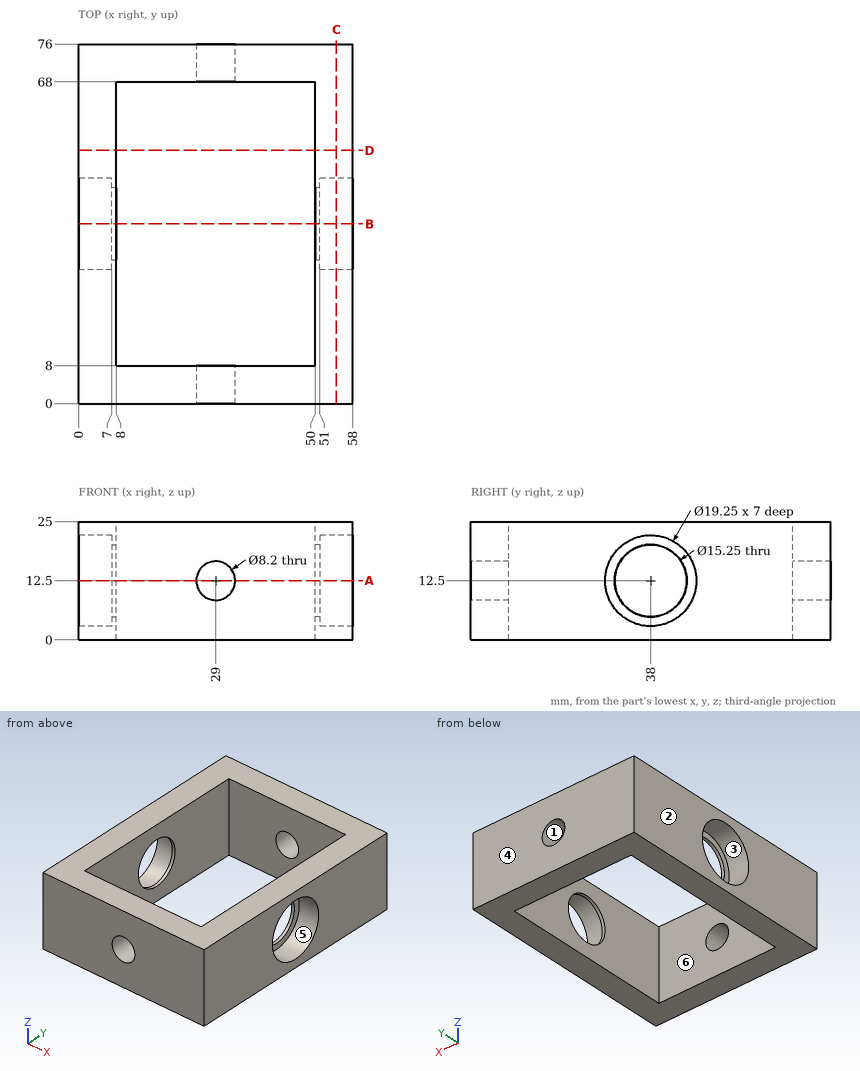
For this review, use the dimensioned drawing (mm, ordinates from the lowest corner) and the shaded views. A direction names the side the tool comes from. Coordinates: 2 decimals unless noted, no trailing zeros. Loops run counter-clockwise (first coordinate to the right, second up) from the corner with the lowest first, then second, coordinate; pieces in that order, holes last. Notation, with made-up numbers: (62, -35) - (66, -35) arc R16 ccw to (66, -4) - close; hole circle Ø5 at (82, -31). An arc over 180 degrees is marked (long way). Use one line per item in the form item = value. Start each with the question number.
1) For pin 1 (6 mm diameter, centred on y = 35, z = 8, fed in from +X); pin 2 (9 mm diameter, centred on y = 38, z = 12.5, fed in from -X), all flat-tipped, find the tip position at first contact; note any pin that passes through.
2) Take a section at A-A (z = 12.5). State how many separate pieces and enclosed holes the cut face has, plus the area to 3 significant figures.
3) To check wall thickness, follow probe 1 along X at (y, z) = (60.5, 3.5); probe 2 along Y at (x, z) = (44, 12.75); probe 3 along Z at (x, y) = (29, 3). State the ranges of each line that lie inside material, in increasing order. Write a range as from..to.
4) Take a section at B-B (y = 38). State the section outline as (x, z) points (3 decimals), plus the area to 3 significant figures.
5) Draft analysis for pull direction X (two halves, no side actions). For the marked faces 1, 2 and 3, state which applies: released by +X, released by -X, zero draft, split by the parting line, or undercut.
6) Take a section at D-D (y = 53.5). State the section outline as (x, z) points, plus the area to 3 significant figures.
7) Take a section at C-C (x = 54.5). State the section outline as (y, z) points (3 decimals).
8) For the marked faces 4, 5 and 6, list the 3-axis set-ups (+Z, -Z, +X, -X, +Y, -Y) from which the entire face can be reached by the end or side of a thin tool; tool diameter is ignored.
From the geometry:
q1.pin_1 = 51
q1.pin_2 = through
q2.separate_pieces = 4
q2.enclosed_holes = 0
q2.area = 1,460 mm2
q3.probe_1 = 0..8, 50..58
q3.probe_2 = 0..8, 68..76
q3.probe_3 = 0..8.4, 16.6..25
q4.outline = (0, 0) - (8, 0) - (8, 4.875) - (7, 4.875) - (7, 2.875) - (0, 2.875) - close; (0, 22.125) - (7, 22.125) - (7, 20.125) - (8, 20.125) - (8, 25) - (0, 25) - close; (50, 0) - (58, 0) - (58, 2.875) - (51, 2.875) - (51, 4.875) - (50, 4.875) - close; (50, 20.125) - (51, 20.125) - (51, 22.125) - (58, 22.125) - (58, 25) - (50, 25) - close
q4.area = 100 mm2
q5.face_1 = undercut
q5.face_2 = released by -X
q5.face_3 = zero draft
q6.outline = (0, 0) - (8, 0) - (8, 25) - (0, 25) - close; (50, 0) - (58, 0) - (58, 25) - (50, 25) - close
q6.area = 400 mm2
q7.outline = (0, 0) - (76, 0) - (76, 25) - (0, 25) - close; hole circle Ø19.25 at (38, 12.5)
q8.face_4 = +Z, -Z, +X, -X, +Y
q8.face_5 = +X
q8.face_6 = +Z, -Z
